```python
from build123d import *

# Parameters (mm, degrees)
BASPROSKE_W         = 4
BASPROSKE_H         = 12
TOOTHCUT_DEPTH      = 18.435595774
TEETHCUTS_COUNT     = 10
TEETHCUTS_ANGLE     = 324
BORSKE_R            = 1
BORE_DEPTH          = 50.0000508
SKETCH_1_W          = 6
SKETCH_1_H          = 6
CUT_EXTRUDE_2_DEPTH = 18.131831434


with BuildPart() as part:
    # BasProSke → Base-Revolve (revolve)
    with BuildSketch(Plane(origin=(0, 0, 0), x_dir=(1, 0, 0), z_dir=(0, 1, 0)), mode=Mode.PRIVATE) as base_revolve_sk:
        with Locations((2, 6)):
            Rectangle(BASPROSKE_W, BASPROSKE_H)
    revolve(base_revolve_sk.sketch.rotate(Axis((-10, 0, 0), (1, 0, 0)), 180), axis=Axis((-10, 0, 0), (1, 0, 0)))

    # TooCutSke → ToothCut (cut, through all)
    with BuildSketch(Plane(origin=(0, 0, 0), x_dir=(0, 0, -1), z_dir=(1, 0, 0))):
        with BuildLine():
            ThreePointArc((1.349961767, 7.376489967), (0, 7.499), (-1.349961767, 7.376489967))
            ThreePointArc((-1.349961767, 7.376489967), (-1.644412889, 9.779161882), (-3.270793922, 11.572041837))
            ThreePointArc((-3.270793922, 11.572041837), (0, 12.0254), (3.270793922, 11.572041837))
            ThreePointArc((3.270793922, 11.572041837), (1.644412889, 9.779161882), (1.349961767, 7.376489967))
        make_face()
    toothcut = extrude(amount=TOOTHCUT_DEPTH, mode=Mode.SUBTRACT)

    # TeethCuts: ToothCut ×10 about axis
    teethcuts_axis = Axis((-10, 0, 0), (1, 0, 0))
    for i in range(1, TEETHCUTS_COUNT):
        add(toothcut.rotate(teethcuts_axis, i * TEETHCUTS_ANGLE / (TEETHCUTS_COUNT - 1)), mode=Mode.SUBTRACT)

    # BorSke → Bore (cut, symmetric)
    with BuildSketch(Plane(origin=(0, 0, 0), x_dir=(0, 0, -1), z_dir=(1, 0, 0))):
        with Locations(Location((0, 0, 0), (0, 0, 180))):
            Circle(BORSKE_R)
    extrude(amount=BORE_DEPTH, both=True, mode=Mode.SUBTRACT)

    # 草图1 → 切除-拉伸2 (cut, through all)
    with BuildSketch(Plane.ZY):
        Rectangle(SKETCH_1_W, SKETCH_1_H)
    extrude(amount=-CUT_EXTRUDE_2_DEPTH, mode=Mode.SUBTRACT)


solid = part.part
```
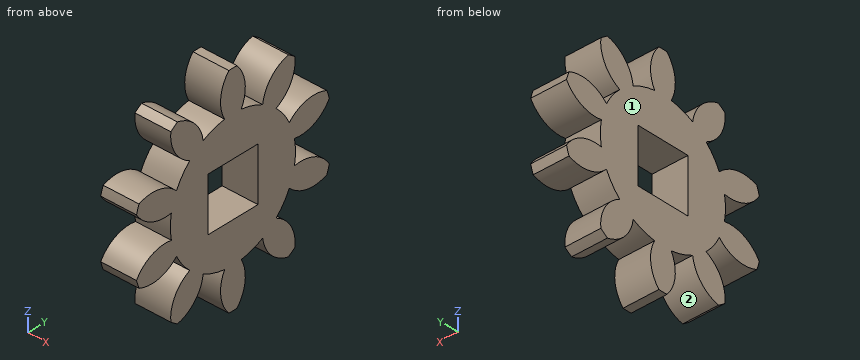
For this review, take the finished solid that the model builds, in its own axes (mm). Face numbers are marked on the shaded views. Give positions to 0.01 mm unless a question says otherwise; leave off trailing zeros. Write each loop counter-clockwise with the first axis right and the second up, starting at its lowest first coordinate (ties: lowest second). Pieces come first, ordered by that corner, then holes.
Item 1: The part is to be moulded in two halves that separate along Y. For the marked faces 1 and 2, say which applies: +Y half, -Y half, draft (parallel to the pull), parting line (faces both ways), or undercut.
Item 2: Take a section at B-B (y = 10.25). Give the boundary of the cut face in (x, z).
Item 3: Take a section at C-C (z = -1). Give the boundary of the cut face in (x, y), and give its area (3 significant figures).
Item 4: Take a section at D-D (z = -6). Give the boundary of the cut face in (x, y), and give its area (3 significant figures).
Item 5: Insertion check: P1, Ø1.2, axis at x = 2.5, z = 0, coming from the -Y side; P2, Ø2, axis at x = 2, z = 1, coming from the +Y side; P3, Ø1.5, axis at x = 2.5, z = -4.5, coming from the -Y side. Each pin has a flat end and moves straight along its axis. Give the tip position at first contact, or say it passes through.
Item 6: Take a section at A-A (z = -8.75). Give the boundary of the cut face in (x, y).
Item 7: Wall thickness on probe 1 along Y at (x, z) = (2.25, -9.5); probe 2 along Y at (x, z) = (3.3, 7.5); probe 3 along Z at (x, y) = (1.9, 6.25): over which ranges is each line inside the solid? List them lowest first.
Established:
1. face 1: draft
1. face 2: undercut
2. outline: (0, -4.45) - (4, -4.45) - (4, -1.9) - (0, -1.9) - close; (0, 1.9) - (4, 1.9) - (4, 4.45) - (0, 4.45) - close
3. outline: (0, -7.43) - (4, -7.43) - (4, -3) - (0, -3) - close; (0, 3) - (4, 3) - (4, 7.43) - (0, 7.43) - close
3. area: 35.5 mm2
4. outline: (0, -6.06) - (4, -6.06) - (4, 6.06) - (0, 6.06) - close
4. area: 48.5 mm2
5. P1: stops at y = -7.5
5. P2: stops at y = 10.4
5. P3: stops at y = -11.4
6. outline: (0, -7.45) - (4, -7.45) - (4, -4.55) - (0, -4.55) - close; (0, -1.44) - (4, -1.44) - (4, 1.44) - (0, 1.44) - close; (0, 4.55) - (4, 4.55) - (4, 7.45) - (0, 7.45) - close
7. probe 1: y = -7.33 to -5.45, -1.48 to 1.48, 5.45 to 7.33
7. probe 2: y = -7.15 to -3.79, -1.03 to 1.03, 3.79 to 7.15
7. probe 3: z = -9.87 to -6.18, -4.14 to 4.14, 6.18 to 9.87
